from build123d import *

# Parameters (mm, degrees)
F0_R     = 6
F0_R_2   = 2.45
F1_DEPTH = 1.5875


with BuildPart() as f1:
    # F0 (on Top) → F1 (new body, symmetric)
    with BuildSketch(Plane.XY):
        Polygon((8.6046455833, -22.0503536392), (15, 0), (1.2463501788, 32.1844235088), (-16.3468942976, 28.3794598042), (-8.6046455833, 22.0503536392), (-15, 0), (-1.2463501788, -32.1844235088), (16.3468942976, -28.3794598042), align=None)
        with Locations((0, -12)):
            Circle(F0_R, mode=Mode.SUBTRACT)
        Circle(F0_R_2, mode=Mode.SUBTRACT)
        with Locations((0, 12)):
            Circle(F0_R, mode=Mode.SUBTRACT)
    extrude(amount=F1_DEPTH, both=True)


solid = f1.part
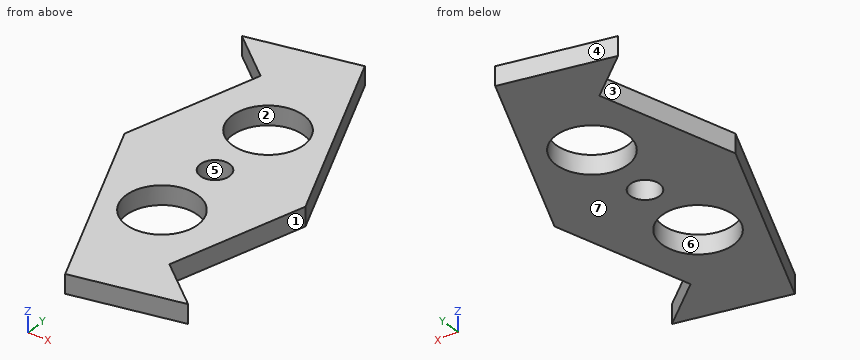
The listing builds one solid part. Answer for the finished solid, in the listing's coordinates (mm). Face numbers are marked on the shaded views. A direction names the side the tool comes from. Round coordinates to 2 decimals unless told otherwise and drop trailing zeros. Loops run counter-clockwise (first coordinate to the right, second up) from the corner with the lowest first, then second, coordinate; pieces in that order, holes last. Notation, with made-up numbers: M -15.5,84 L 14.5,84 A30 ccw 14.5,107 Z; hole C 21,37.5 d4. An arc over 180 degrees is marked long. Write each question's results on one line, items separated by ' | '. Start each with the question number.
1) Which of the six approach directions +Z, -Z, +X, -X, +Y, -Y give full straight-line access (tool end or side, diameter ignored) to the marked faces 1, 2 and 3?
2) Find section A-A on y = -7. Write down the section's boundary in (x, z), plus the area to 3 significant figures.
3) Straight lines are drawn through the part: probe 1 along Y at (x, z) = (-3.5, -0.95); probe 2 along Y at (x, z) = (2, 0.6); probe 3 along Y at (x, z) = (0, 0.5). For each, find the intervals that lie inside material, in ascending order.
4) Find section B-B on z = 0.15. Write down the section's boundary in (x, y), plus the area to 3 significant figures.
5) Find section D-D on y = 12. Write down the section's boundary in (x, z).
6) Each of these flat-tipped pins is pushed along its axis until it touches: pin 1 (1 mm diameter, centred on y = -24, z = 1, fed in from -X); pin 2 (1 mm diameter, centred on y = -11.5, z = 1, fed in from +X); pin 3 (4.5 mm diameter, centred on x = 0, y = 0, fed in from +Z); pin 4 (1.5 mm diameter, centred on y = -3, z = 1, fed in from -X). Where does it stop, or does it pass through?
7) Find section C-C on x = 0. Write down the section's boundary in (y, z).
8) Determine the mould class of the marked faces 4, 5, 6 and 7 for opening direction X: pulls with the +X half, pulls with the -X half, needs draft (parallel to the pull), parting line crosses it, or undercut.
Final values:
1) face 1: +Z, -Z, +X | face 2: +Z, -Z | face 3: +Z, -Z, -X
2) outline: M -12.01,-1.59 L -3.32,-1.59 L -3.32,1.59 L -12.01,1.59 Z; M 3.32,-1.59 L 12.97,-1.59 L 12.97,1.59 L 3.32,1.59 Z | area: 58.2 mm²
3) probe 1: -26.91 to -16.87, -7.13 to 7.13, 16.87 to 31.16 | probe 2: -31.48 to -17.66, -6.34 to -1.42, 1.42 to 6.34, 17.66 to 30.42 | probe 3: -31.91 to -18, -6 to -2.45, 2.45 to 6, 18 to 31.91
4) outline: M -16.35,28.38 L -8.6,22.05 L -15,0 L -1.25,-32.18 L 16.35,-28.38 L 8.6,-22.05 L 15,0 L 1.25,32.18 Z; hole C 0,-12 d12; hole C 0,12 d12; hole C 0,0 d4.9 | area: 1,010 mm²
5) outline: M -11.52,-1.59 L -6,-1.59 L -6,1.59 L -11.52,1.59 Z; M 6,-1.59 L 9.87,-1.59 L 9.87,1.59 L 6,1.59 Z
6) pin 1: x = -4.96 | pin 2: x = 11.81 | pin 3: through | pin 4: x = -14.04
7) outline: M -31.91,-1.59 L -18,-1.59 L -18,1.59 L -31.91,1.59 Z; M -6,-1.59 L -2.45,-1.59 L -2.45,1.59 L -6,1.59 Z; M 2.45,-1.59 L 6,-1.59 L 6,1.59 L 2.45,1.59 Z; M 18,-1.59 L 31.91,-1.59 L 31.91,1.59 L 18,1.59 Z
8) face 4: pulls with the -X half | face 5: undercut | face 6: undercut | face 7: needs draft
